The listing builds one solid part. Answer for the finished solid, in the listing's coordinates (mm). A direction names the side the tool comes from. Give positions to 0.01 mm unless a question says otherwise; leave off trailing zeros. Order: outer loops, then holes, each group sorted by start corner. A loop starts at its lowest first (then second) coordinate and runs counter-clockwise, first axis right, second up. Notation, with made-up numbers: (75.25, 41) -> (81.25, 41) arc R7 cw to (81.25, 51) -> close; hole circle Ø6 at (81, -11.75). An arc over 180 degrees is marked (long way). One line per question, with ' | ' between items. Start each with the question number.
```python
from build123d import *

# Parameters (mm, degrees)
CROQUIS1_W              = 24
CROQUIS1_H              = 5
SALIENTE_EXTRUIR1_DEPTH = 1.5
MATRIZC1_COUNT          = 10
CROQUIS3_R              = 4
CORTAR_EXTRUIR1_DEPTH   = 1
CROQUIS4_R              = 2.5
CORTAR_EXTRUIR2_DEPTH   = 5
SCALE1_SCALE            = 0.957142857


with BuildPart() as part:
    # Croquis1 → Revolución1 (revolve)
    with BuildSketch(Plane.XY):
        Polygon((-12, 26.5), (-12, 30), (-11, 30), (-11, 28.33342991), (12, 28.33342991), (12, 30), (13, 30), (13, 26.5), (5.499345391, 26.5), (5.499345391, 25), (-5.499345391, 25), align=None)
        with Locations((-5, 2.5)):
            Rectangle(CROQUIS1_W, CROQUIS1_H)
    revolve(axis=Axis((-17, 0, 0), (-1, 0, 0)))

    # Croquis2 → Saliente-Extruir1 (add, symmetric)
    with BuildSketch(Plane.XY):
        with BuildLine():
            Line((13, 26.5), (13, 23.5))
            add(Edge.make_bspline(
                [(13, 23.5), (12.190614948, 13.316000856), (7, 4.7)],
                knots=[0, 0, 0, 1, 1, 1], degree=2))
            Line((7, 4.7), (5.499345391, 4.7))
            Line((5.499345391, 4.7), (5.499345391, 26.5))
            Line((5.499345391, 26.5), (13, 26.5))
        make_face()
    saliente_extruir1 = extrude(amount=SALIENTE_EXTRUIR1_DEPTH, both=True)

    # MatrizC1: Saliente-Extruir1 ×10 about axis
    matrizc1_axis = Axis((5.499345391, 0, 0), (1, 0, 0))
    for i in range(1, MATRIZC1_COUNT):
        add(saliente_extruir1.rotate(matrizc1_axis, i * 360 / MATRIZC1_COUNT))

    # Croquis3 → Cortar-Extruir1 (cut)
    with BuildSketch(Plane(origin=(7, 0, 0), x_dir=(0, 0, -1), z_dir=(1, 0, 0))):
        with Locations(Location((0, 0, 0), (0, 0, 90))):
            Circle(CROQUIS3_R)
    extrude(amount=-CORTAR_EXTRUIR1_DEPTH, mode=Mode.SUBTRACT)

    # Croquis4 → Cortar-Extruir2 (cut)
    with BuildSketch(Plane.ZY.offset(17)):
        with Locations(Location((0, 0, 0), (0, 0, 270))):
            Circle(CROQUIS4_R)
    extrude(amount=-CORTAR_EXTRUIR2_DEPTH, mode=Mode.SUBTRACT)


with BuildPart() as part_1:
    # Scale1: scaled about (1.224671263, 0, 0)
    add(part.part.scale(SCALE1_SCALE).moved(Location((0.052485911, 0, 0))))


solid = part_1.part
```
(1) Determine the mould class of faces 1 (the face through (8.855, -24.094, -7.925)), 2 (the face through (8, 17, 1.436)), 3 (the face through (-10.95, -22.79, 17.47)) for opening direction Z: pulls with the +Z half, pulls with the -Z half, needs draft (parallel to the pull), parting line crosses it, or undercut.
(2) Given P1, Ø10, axis at x = -6, y = -2.5, coming from the -Z side; P2, Ø6, axis at y = 1.5, z = 1.5, coming from the +X side; P3, Ø9.5, axis at y = -4.5, z = -9, coming from the -X side; P4, Ø4, axis at y = 14.5, z = -6, coming from the -X side, each flat-ended and moving along its own axis, determine where each tip first touches the part or whether it passes through.
(3) Consider line 1 (Y direction, x = -2.25, z = 0); line 2 (X direction, y = -25, z = 13). Determine where each line is inside the solid, lowest interval first.
(4) For faces 4 (the face through (-0.02, -5.19, 23.36)), 5 (the face through (8.16, 4, -16.96)), determine the directions among +Z, -Z, +X, -X, +Y, -Y from which every point of the face is accessible in a straight line to the end or side of a thin tool.
(5) The part is cut by section B-B on z = 6. State how many separate pieces and enclosed holes the cut face has, plus the area to 3 significant figures.
(6) The part is cut by section A-A on x = 3. Determine the outline of the cut face in (y, z), plus the area to 3 significant figures.
Result sheet:
1) face 1: undercut | face 2: undercut | face 3: parting line crosses it
2) P1: stops at z = -28.71 | P2: stops at x = 7.11 | P3: stops at x = 5.32 | P4: passes through
3) line 1: y = -27.12 to -23.93, -4.79 to 4.79, 23.93 to 27.12 | line 2: x = -11.43 to -10.48, 11.54 to 12.5
4) face 4: -X | face 5: +X
5) separate pieces: 6 | enclosed holes: 0 | area: 190 mm^2
6) outline: circle Ø54.24 at (0, 0); circle Ø9.57 at (0, 0); hole circle Ø47.86 at (0, 0) | area: 584 mm^2
